Can you work these out from the model? Positions are in its coordinate system, mm. A direction names the side the tool comes from. Coordinates: 2 decimals unless noted, no trailing zeros. Order: outer loops, then holes, each group sorted by start corner. A loop starts at its lowest first (then second) coordinate and runs counter-clockwise, first axis right, second up. Notation, with made-up numbers: (42.5, -28) -> (80.5, -28) arc R15 ccw to (80.5, -23) -> close; hole circle Ø11 at (73.5, 40). An arc over 180 degrees is marked (long way). Answer in a Markdown table with one row per item.
```python
from build123d import *

# Parameters (mm, degrees)
SKIZZE3_W                            = 190
SKIZZE3_H                            = 6
AUFSATZ_LINEAR_AUSTRAGEN2_DEPTH      = 55
AUFSATZ_LINEAR_AUSTRAGEN2_DEPTH_BACK = 55
SCHNITT_LINEAR_AUSTRAGEN5_DEPTH      = 169.5
OUTLINETOP_R                         = 3
SCHNITT_LINEAR_AUSTRAGEN6_DEPTH      = 169.5
SKIZZE8_W                            = 39.137679275
SKIZZE8_H                            = 43
SCHNITT_LINEAR_AUSTRAGEN7_DEPTH      = 169.5
SKIZZE9_R                            = 4
SCHNITT_LINEAR_AUSTRAGEN8_DEPTH      = 169.5


with BuildPart() as part:
    # Skizze3 → Aufsatz-Linear austragen2 (new body, two sides)
    with BuildSketch(Plane(origin=(0, 0, 0), x_dir=(0, 0, -1), z_dir=(1, 0, 0))) as aufsatz_linear_austragen2_sk:
        with Locations((-190, 166.5)):
            Rectangle(SKIZZE3_W, SKIZZE3_H)
    extrude(amount=AUFSATZ_LINEAR_AUSTRAGEN2_DEPTH)
    extrude(aufsatz_linear_austragen2_sk.sketch, amount=-AUFSATZ_LINEAR_AUSTRAGEN2_DEPTH_BACK)

    # Holes → Schnitt-Linear austragen5 (cut)
    with BuildSketch(Plane(origin=(0, 0, 0), x_dir=(1, 0, 0), z_dir=(0, 1, 0))):
        with BuildLine():
            ThreePointArc((-19.706276733, -148.936330777), (-23.210222992, -150.810105621), (-26.537525439, -152.982139225))
            ThreePointArc((-26.537525439, -152.982139225), (-27.342866764, -157.865931333), (-22.459074657, -158.671272659))
            ThreePointArc((-22.459074657, -158.671272659), (-19.643132597, -156.833050591), (-16.677694436, -155.247249036))
            ThreePointArc((-16.677694436, -155.247249036), (-15.036526455, -150.577498758), (-19.706276733, -148.936330777))
        make_face()
        with BuildLine():
            ThreePointArc((44.855396174, -182.090783424), (43.995374204, -178.211475011), (42.800520871, -174.421884392))
            ThreePointArc((42.800520871, -174.421884392), (38.314526197, -172.330030721), (36.222672526, -176.816025395))
            ThreePointArc((36.222672526, -176.816025395), (37.23389342, -180.023208327), (37.961741903, -183.306320668))
            ThreePointArc((37.961741903, -183.306320668), (42.01633766, -186.145379182), (44.855396174, -182.090783424))
        make_face()
        with BuildLine():
            ThreePointArc((-8.120828878, -234.817568107), (-4.183818236, -235.354800603), (-0.214966211, -235.546855679))
            ThreePointArc((-0.214966211, -235.546855679), (3.301513476, -232.063413328), (-0.181928876, -228.546933641))
            ThreePointArc((-0.181928876, -228.546933641), (-3.540823214, -228.384394775), (-6.872769749, -227.929727487))
            ThreePointArc((-6.872769749, -227.929727487), (-10.940719624, -230.749618233), (-8.120828878, -234.817568107))
        make_face()
    extrude(amount=SCHNITT_LINEAR_AUSTRAGEN5_DEPTH, mode=Mode.SUBTRACT)

    # OutlineTop → Schnitt-Linear austragen6 (cut)
    with BuildSketch(Plane(origin=(0, 0, 0), x_dir=(1, 0, 0), z_dir=(0, 1, 0))):
        with Locations((-15, -270)):
            Circle(OUTLINETOP_R)
        with Locations((15, -270)):
            Circle(OUTLINETOP_R)
        with Locations((-15, -110)):
            Circle(OUTLINETOP_R)
        with Locations((15, -110)):
            Circle(OUTLINETOP_R)
    extrude(amount=SCHNITT_LINEAR_AUSTRAGEN6_DEPTH, mode=Mode.SUBTRACT)

    # Skizze8 → Schnitt-Linear austragen7 (cut)
    with BuildSketch(Plane(origin=(0, 0, 0), x_dir=(1, 0, 0), z_dir=(0, 1, 0))):
        with Locations((-35.431160363, -230.5)):
            Rectangle(SKIZZE8_W, SKIZZE8_H)
    extrude(amount=SCHNITT_LINEAR_AUSTRAGEN7_DEPTH, mode=Mode.SUBTRACT)

    # Skizze9 → Schnitt-Linear austragen8 (cut)
    with BuildSketch(Plane(origin=(0, 0, 0), x_dir=(1, 0, 0), z_dir=(0, 1, 0))):
        with Locations((-15, -110)):
            Circle(SKIZZE9_R)
        with Locations((15, -110)):
            Circle(SKIZZE9_R)
        with Locations((15, -270)):
            Circle(SKIZZE9_R)
        with Locations((-15, -270)):
            Circle(SKIZZE9_R)
    extrude(amount=SCHNITT_LINEAR_AUSTRAGEN8_DEPTH, mode=Mode.SUBTRACT)


solid = part.part
```
(1) Suppose I cut it at D-D (x = 15). Please give me the cut outline in (y, z).
Response values:
| item | result |
|---|---|
| outline | (163.5, 95) -> (169.5, 95) -> (169.5, 106) -> (163.5, 106) -> close; (163.5, 114) -> (169.5, 114) -> (169.5, 266) -> (163.5, 266) -> close; (163.5, 274) -> (169.5, 274) -> (169.5, 285) -> (163.5, 285) -> close |
(2) Will this pin go through, and if not, where does the flat tip stop? pin 1 Ø1 at (y, z) = (164, 231) entering from -X.
Response values:
| item | result |
|---|---|
| pin 1 | x = -15.86 |
(3) On a 3-axis mill with a long thin cutter (end or side, diameter ignored), from which of +Z, -Z, +X, -X, +Y, -Y can I reach the whole of each face in a straight line? I mean faces 1 (the flat face through (1, 166, 95)), 2 (the flat face through (-15.862, 166, 231)), 3 (the cylindrical face through (-4.24, 166.46, 235.35)). Say none if no direction works.
Response values:
| item | result |
|---|---|
| face 1 | -Z, +X, -X, +Y, -Y |
| face 2 | -X, +Y, -Y |
| face 3 | +Y, -Y |
(4) Suppose I cut it at C-C (y = 166.7). Please give me the cut outline in (x, z).
Response values:
| item | result |
|---|---|
| outline | (-55, 95) -> (55, 95) -> (55, 285) -> (-55, 285) -> (-55, 252) -> (-15.86, 252) -> (-15.86, 209) -> (-55, 209) -> close; hole (-26.54, 152.98) arc R45.55 ccw to (-19.71, 148.94) arc R3.5 ccw to (-16.68, 155.25) arc R38.55 cw to (-22.46, 158.67) arc R3.5 ccw to start; hole circle Ø8 at (-15, 110); hole circle Ø8 at (-15, 270); hole (-8.12, 234.82) arc R3.5 ccw to (-6.87, 227.93) arc R38.55 cw to (-0.18, 228.55) arc R3.5 ccw to (-0.21, 235.55) arc R45.55 ccw to start; hole circle Ø8 at (15, 110); hole circle Ø8 at (15, 270); hole (36.22, 176.82) arc R3.5 ccw to (42.8, 174.42) arc R45.55 ccw to (44.86, 182.09) arc R3.5 ccw to (37.96, 183.31) arc R38.55 cw to start |
(5) Suppose I cut it at A-A (x = -38). Please give me the cut outline in (y, z), and give its area (3 significant figures).
Response values:
| item | result |
|---|---|
| outline | (163.5, 95) -> (169.5, 95) -> (169.5, 209) -> (163.5, 209) -> close; (163.5, 252) -> (169.5, 252) -> (169.5, 285) -> (163.5, 285) -> close |
| area | 882 mm2 |
(6) I need wall thicknesses on line 1 (X direction, y = 165.85, z = 110); line 2 (Z direction, x = 15, y = 167.2); line 3 (Z direction, x = -16, y = 164.3). Which ranges of each line are inside material? Lowest first, please. Write a range as [from, to].
Response values:
| item | result |
|---|---|
| line 1 | [-55, -19], [-11, 11], [19, 55] |
| line 2 | [95, 106], [114, 266], [274, 285] |
| line 3 | [95, 106.13], [113.87, 149.36], [154.82, 209], [252, 266.13], [273.87, 285] |
(7) Suppose I cut it at B-B (z = 110). Please give me the cut outline in (x, y), and give its area (3 significant figures).
Response values:
| item | result |
|---|---|
| outline | (-55, 163.5) -> (-19, 163.5) -> (-19, 169.5) -> (-55, 169.5) -> close; (-11, 163.5) -> (11, 163.5) -> (11, 169.5) -> (-11, 169.5) -> close; (19, 163.5) -> (55, 163.5) -> (55, 169.5) -> (19, 169.5) -> close |
| area | 564 mm2 |
(8) We'd pull the mould along X, two halves only. Please class faces 4 (the flat face through (1, 166, 285)), 5 (the cylindrical face through (-23.16, 166.46, 150.78)), 6 (the flat face through (55, 167, 191)): +X half, -X half, draft (parallel to the pull), parting line (faces both ways), or undercut.
Response values:
| item | result |
|---|---|
| face 4 | draft |
| face 5 | undercut |
| face 6 | +X half |
